Model file for the job. Use its own axes, mm. A direction names the side the tool comes from. Give positions to 0.01 mm unless a question says otherwise; leave off trailing zeros. One line per item, written item: value. Start each with the question number.
(1) Probe L1, parallel to Y at x = 5.25, z = 10; L2, parallel to Y at x = 3.5, z = 0; L3, parallel to Y at x = 2.75, z = 0. List the from-to ranges inside material, lowest first.
(2) 3-axis set-ups, long thin cutter, end or side, ignore diameter. For faces 1 (the face through (10.29, -3.65, -0.13)), 2 (the face through (0, -18, -6)), 3 (the face through (6.2, 0.1, -9.5)): which of +Z, -Z, +X, -X, +Y, -Y reach the whole face in a straight line?
(3) Drop flat-ended pins along their axis: P1, Ø15, axis at y = 2, z = 1.5, coming from the -X side; P2, Ø6.5, axis at y = 2, z = 3, coming from the -X side; P3, Ø3, axis at x = 7, y = 17, coming from the -Z side. Give the stop position or say it passes through.
(4) Cut at A-A, the plane x = 4.75. State how many separate pieces and enclosed holes the cut face has, and give its area (3 significant figures).
(5) Mould opens along Y. For faces 4 (the face through (4.084, 18.597, -4.13)), 5 (the face through (6.2, 7, -17)), 6 (the face through (1.6, 19.2, -0.1)) say: pulls with the +Y half, pulls with the -Y half, needs draft (parallel to the pull), parting line crosses it, or undercut.
from build123d import *
from build123d.topology import SkipClean

# Parameters (mm, degrees)
SKETCH3_R               = 9.5
BOSS_EXTRUDE1_DEPTH     = 16
CUT_EXTRUDE1_DEPTH      = 21.892582416
CUT_EXTRUDE1_DEPTH_BACK = 21.892582416
SHELL7_T                = -0.3
SKETCH8_R               = 10.705762979
CUT_EXTRUDE5_DEPTH      = 10
CUT_EXTRUDE6_DEPTH      = 30


with BuildPart() as part:
    # Sketch3 → Boss-Extrude1 (new body)
    with BuildSketch(Plane.ZY):
        Circle(SKETCH3_R)
    extrude(amount=-BOSS_EXTRUDE1_DEPTH)

    # Sketch4 → Cut-Extrude1 (cut, two sides: drawn at the far end of the back side and taken through both)
    with BuildSketch(Plane.XY.offset(-CUT_EXTRUDE1_DEPTH_BACK)):
        Polygon((2.5, 9.5), (18.05891099, 17.267926144), (18.05891099, -17.267926144), (2.5, -9.5), (16, 0), align=None)
    extrude(amount=CUT_EXTRUDE1_DEPTH + CUT_EXTRUDE1_DEPTH_BACK, mode=Mode.SUBTRACT)

    # Shell7
    shell7_openings = [part.faces().sort_by_distance(p)[0] for p in [
        (0, 0, 0),
    ]]
    offset(amount=SHELL7_T, openings=shell7_openings, kind=Kind.INTERSECTION)

    # Sketch1 → Revolve1 (revolve)
    with SkipClean():  # the faces are left unmerged after this step: merging them gives an invalid solid
        with BuildSketch(Plane.XY, mode=Mode.PRIVATE) as revolve1_sk:
            Polygon((0, 18.75), (0, 21.75), (1.6, 21.75), (1.6, 19.05), (6.5, 19.05), (6.5, 17.65), (2.5, 12.5), (2.5, 9.5), (2.2, 9.5), (2.2, 12.602819589), (6.2, 17.752819589), (6.2, 18.75), align=None)
        revolve(revolve1_sk.sketch.rotate(Axis((0, 0, 0), (1, 0, 0)), 90), axis=Axis((0, 0, 0), (1, 0, 0)))

    # Sketch8 → Cut-Extrude5 (cut)
    with SkipClean():  # the faces are left unmerged after this step: merging them gives an invalid solid
        with BuildSketch(Plane.ZY.offset(-2.2)):
            Circle(SKETCH8_R)
        extrude(amount=CUT_EXTRUDE5_DEPTH, mode=Mode.SUBTRACT)

    # Sketch9 → Cut-Extrude6 (cut)
    with SkipClean():  # the faces are left unmerged after this step: merging them gives an invalid solid
        with BuildSketch(Plane.ZY.offset(-2.2)):
            with BuildLine():
                Line((-9.2, -0.01), (9.2, -0.01))
                ThreePointArc((9.2, -0.01), (9.200005435, 0), (9.2, 0.01))
                Line((9.2, 0.01), (-9.2, 0.01))
                ThreePointArc((-9.2, 0.01), (-9.200005435, 0), (-9.2, -0.01))
            make_face()
        extrude(amount=-CUT_EXTRUDE6_DEPTH, mode=Mode.SUBTRACT)


solid = part.part
Answers follow:
1. L1: y = -16.21 to -15.86, -13.16 to -12.54, 12.54 to 13.16, 15.86 to 16.21
1. L2: y = -19.05 to -18.75, -14.28 to -13.79, -8.8 to -8.43, 8.43 to 8.8, 13.79 to 14.28, 18.75 to 19.05
1. L3: y = -19.05 to -18.75, -13.31 to -12.82, -9.32 to -8.96, 8.96 to 9.32, 12.82 to 13.31, 18.75 to 19.05
2. face 1: -X
2. face 2: +Z, -Z, -X, +Y, -Y
2. face 3: +X
3. P1: stops at x = 2.2
3. P2: stops at x = 8.02
3. P3: stops at z = -10.95
4. separate pieces: 3
4. enclosed holes: 3
4. area: 102 mm²
5. face 4: parting line crosses it
5. face 5: undercut
5. face 6: needs draft
